Input: part model. Units: mm. Frame: model coordinates. Face numbers are marked on the shaded views. A direction names the side the tool comes from. Coordinates: 2 decimals unless noted, no trailing zeros. Write each loop counter-clockwise with the first axis right and the second up, starting at its lowest first coordinate (ties: lowest second). Pieces come first, ordered by that corner, then holes. Notation, with made-up numbers: (45.5, 58.25) - (53.5, 58.25) arc R19 cw to (53.5, 63.25) - close; hole circle Ø8 at (79, -35). An arc over 180 degrees is marked (long way). One line per question, with ' | ' between items. Start each with the question number.
1) Line query: line 1 (Z direction, x = 2.5, y = 6.75); line 2 (Z direction, x = 10, y = 5.5); line 3 (Y direction, x = 10, z = -37.5). Output: solid intervals per line, ascending.
2) Reachability of the marked faces 1, 2 and 3 from +Z, -Z, +X, -X, +Y, -Y: full face, straight path, thin tool, end or side. Return the list, or none.
3) Section query C-C on x = 11.5. Return loops of the section in (y, z), and give its area (3 significant figures).
4) Section query A-A on y = 8.75. Return loops of the section in (x, z).
5) First-contact query: P1, Ø3.5, axis at y = 18, z = -4.5, coming from the -X side; P2, Ø4, axis at x = 10.5, z = -16, coming from the +Y side; P3, Ø1, axis at x = 4, z = -23.5, coming from the +Y side. Flat tips, straight axial feed; report the tip coordinate or a pass-through.
6) Draft query along Z for the marked faces 4, 5 and 6. Return one class per face: released by +Z, released by -Z, zero draft, split by the parting line, or undercut.
7) Section query D-D on y = 18.75. Return loops of the section in (x, z), and give its area (3 significant figures).
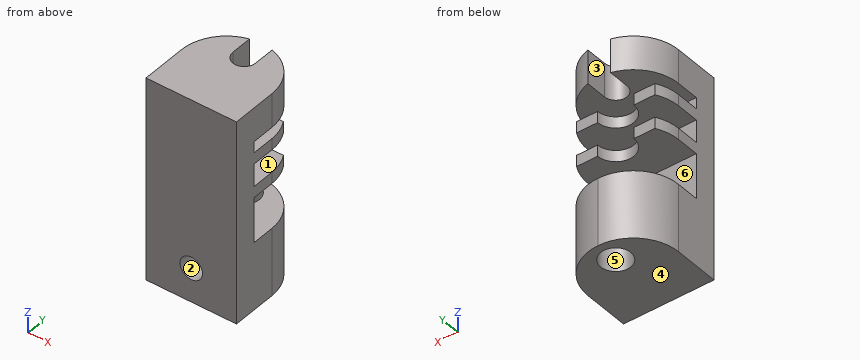
Autodesk Inventor part; units mm, degrees
ref_plane "YZ Plane" through (0, 0, 0) normal (1, 0, 0) x (0, 1, 0)
ref_plane "XZ Plane" through (0, 0, 0) normal (0, 1, 0) x (-1, 0, 0)
ref_plane "XY Plane" through (0, 0, 0) normal (0, 0, 1) x (1, 0, 0)
sketch "Sketch1" plane through (0, 0, 0) normal (0, 0, 1) x (1, 0, 0)
  line L0 (0, 20) -> (20, 20)
  line L1 (20, 20) -> (20, 0)
  line L2 (20, 0) -> (0, 0)
  line L3 (0, 0) -> (0, 20)
  dimension "d0" = 20
  dimension "d1" = 20
extrude "Extrusion1" add sketch "Sketch1" against normal blind 45
fillet "Fillet1" radius 10 2 edges at (0, 20, -22.5) (20, 20, -22.5)
sketch "Sketch2" plane through (20, 0, 0) normal (1, 0, 0) x (0, 0, -1)
  line L0 (20, 21) -> (30, 21)
  line L1 (30, 21) -> (30, 5)
  line L2 (30, 5) -> (20, 5)
  line L3 (20, 5) -> (20, 21)
  line L4 (12.5, 21) -> (17.5, 21)
  line L5 (17.5, 21) -> (17.5, 5)
  line L6 (17.5, 5) -> (12.5, 5)
  line L7 (12.5, 5) -> (12.5, 21)
  line L8 (7.5, 21) -> (10, 21)
  line L9 (10, 21) -> (10, 5)
  line L10 (10, 5) -> (7.5, 5)
  line L11 (7.5, 5) -> (7.5, 21)
  line L12 (45, 10) -> (45, 0)
  line L13 (0, 0) -> (45, 0)
  point P0 (25, 5)
  dimension "d5" = 15
  dimension "d6" = 25
  dimension "d7" = 27.5
  dimension "d8" = 32.5
  dimension "d9" = 35
  dimension "d10" = 37.5
  dimension "d11" = 5
  dimension "d12" = 21
extrude "Extrusion2" cut sketch "Sketch2" against normal blind 45
sketch "Sketch3" plane through (20, 0, 0) normal (1, 0, 0) x (0, 0, -1)
  line L0 (9.5, 21) -> (20.5, 21)
  line L1 (20.5, 21) -> (20.5, 15)
  line L2 (20.5, 15) -> (9.5, 15)
  line L3 (9.5, 15) -> (9.5, 21)
  line L4 (0, 0) -> (45, 0)
  line L5 (10, 10) -> (10, 20)
  line L6 (20, 20) -> (20, 10)
  point P0 (15, 15)
  dimension "d15" = 15
  dimension "d16" = 6
  dimension "d17" = 0.5
  dimension "d18" = 0.5
extrude "Extrusion3" cut sketch "Sketch3" against normal blind 45
sketch "Sketch4" plane through (0, 0, -45) normal (0, 0, -1) x (-1, 0, 0)
  circle A0 centre (-10, 15) radius 2
  line L0 (-20, 0) -> (0, 0)
  arc A1 (0, 10) -> (-20, 10) centre (-10, 10) ccw
  point P0 (-10, 20)
  dimension "d21" = 4
  dimension "d22" = 15
hole "Hole1" at (10, 15, -45) direction (0, 0, 1) diameter 6.647 depth 25
sketch "Sketch5" plane through (0, 0, 0) normal (0, 0, 1) x (1, 0, 0)
  circle A0 centre (10, 15) radius 3.3235
  arc A1 (7.5, 15) -> (12.5, 15) centre (10, 15) ccw
  line L0 (7.5, 21) -> (12.5, 21)
  line L1 (12.5, 21) -> (12.5, 15)
  line L2 (7.5, 15) -> (7.5, 21)
  point P0 (0, 0)
  dimension "d31" = 5
  dimension "d32" = 2.5
  dimension "d33" = 2.5
  dimension "d34" = 6
extrude "Extrusion4" cut sketch "Sketch5" against normal up to surface (10 mm away) contours L1 A1 L2 A0 | A0 L2 L0 L1 picked at (9.8656, 16.0996)
sketch "Sketch6" plane through (20, 5, -20) normal (0, 0, -1) x (-1, 0, 0)
  arc A0 (7.5, 10) -> (12.5, 10) centre (10, 10) ccw
  circle A1 centre (10, 10) radius 4
  point P0 (20, -5)
  dimension "d37" = 8
extrude "Extrusion5" cut sketch "Sketch6" against normal up to surface (12.5 mm away)
sketch "Sketch7" plane through (0, 0, 0) normal (0, -1, 0) x (1, 0, 0)
  circle A0 centre (10, -37.5) radius 2.5
  line L0 (20, -45) -> (0, -45)
  point P0 (0, 0)
  point P1 (10, -45)
  dimension "d40" = 5
  dimension "d41" = 7.5
extrude "Extrusion6" cut sketch "Sketch7" against normal blind 10
properties part number "Extractor Body"
Answer key:
1) line 1: -45 to -30, -20 to -17.5, -12.5 to -10, -7.5 to 0 | line 2: -45 to -40, -35 to -30, -20 to -17.5, -12.5 to -10, -7.5 to 0 | line 3: 10 to 11.68, 18.32 to 20
2) face 1: +X, -X, +Y | face 2: -Y | face 3: +Z, +Y
3) outline: (0, -45) - (12.03, -45) - (12.03, -30) - (5, -30) - (5, -20) - (11.29, -20) - (11.29, -17.5) - (5, -17.5) - (5, -12.5) - (11.29, -12.5) - (11.29, -10) - (5, -10) - (5, -7.5) - (13, -7.5) - (13, 0) - (0, 0) - (0, -35.5) - (10, -35.5) - (10, -39.5) - (0, -39.5) - close; (17.97, -45) - (19.89, -45) - (19.89, -30) - (17.97, -30) - close | area: 411 mm²
4) outline: (0, -45) - (20, -45) - (20, -30) - (0, -30) - close; (0, -20) - (20, -20) - (20, -17.5) - (0, -17.5) - close; (0, -12.5) - (20, -12.5) - (20, -10) - (0, -10) - close; (0, -7.5) - (20, -7.5) - (20, 0) - (0, 0) - close; hole circle Ø5 at (10, -37.5)
5) P1: x = 2.19 | P2: y = 11.44 | P3: y = 5
6) face 4: released by -Z | face 5: zero draft | face 6: undercut
7) outline: (5.16, -45) - (14.84, -45) - (14.84, -30) - (5.16, -30) - close; (5.16, -7.5) - (7.5, -7.5) - (7.5, 0) - (5.16, 0) - close; (12.5, -7.5) - (14.84, -7.5) - (14.84, 0) - (12.5, 0) - close | area: 180 mm²
